Here's how the part is built. I have some questions about the finished solid (model axes, mm). Face numbers are marked on the shaded views. A direction names the side the tool comes from. Round coordinates to 2 decimals unless told otherwise and drop trailing zeros. Loops run counter-clockwise (first coordinate to the right, second up) from the corner with the lowest first, then second, coordinate; pieces in that order, holes last. Notation, with made-up numbers: M 68,12.25 L 75,12.25 A14 ccw 75,22.25 Z; hole C -30,26 d3. An arc over 180 degrees is marked long. One line per question, with ' | ' between items. Start each with the question number.
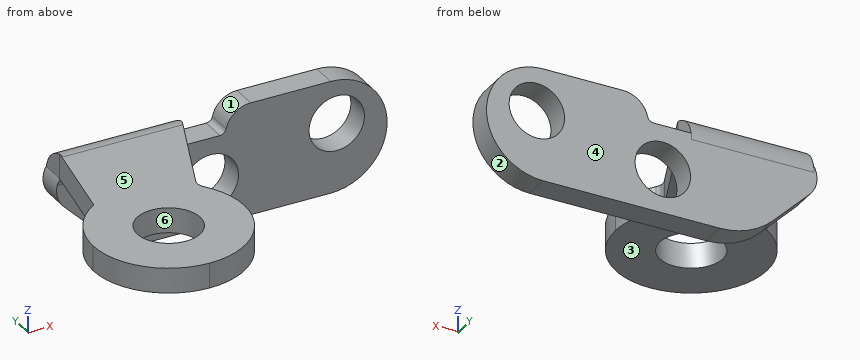
```python
from build123d import *

# Parameters (mm, degrees)
F1_DEPTH     = 2
F2_D         = 4.4
F3_W         = 13.8216872486
F3_H         = 2
F4_DEPTH     = 20.5
F5_R         = 2.5
F6_DEPTH     = 25
F7_R         = 1
F8_T4_DEPTH  = 12.2216872486
F8_T10_DEPTH = 12.2216872486
F8_S11_R     = 2
F8_T12_DEPTH = 8
F10_DEPTH    = 9.7216872486


# Not quite as in the source:
# - a fillet or chamfer that OpenCascade refuses, or shapes differently, is made with other operations: its cross-section is extruded or revolved along the edge and cut away or added


with BuildPart() as f1:
    # F0 (on Front) → F1 (new body)
    with BuildSketch(Plane.XZ):
        with BuildLine():
            Line((-5.5351668461, -4.5), (8.4648331539, -4.5))
            ThreePointArc((8.4648331539, -4.5), (12.9648331539, 0), (8.4648331539, 4.5))
            Line((8.4648331539, 4.5), (2.1292536968, 4.5))
            ThreePointArc((2.1292536968, 4.5), (0.8745117295, 4.0574410408), (0.1750670613, 2.9256225954))
            ThreePointArc((0.1750670613, 2.9256225954), (0.0002058943, 2.6426679841), (-0.3134795975, 2.5320282443))
            Line((-0.3134795975, 2.5320282443), (-13.0351668461, 2.5320282443))
            ThreePointArc((-13.0351668461, 2.5320282443), (-13.2536814771, 1.2929397336), (-12.6890072408, 0.1685590205))
            Line((-12.6890072408, 0.1685590205), (-9.7778075332, -2.7426406871))
            ThreePointArc((-9.7778075332, -2.7426406871), (-7.8312674403, -4.0432771951), (-5.5351668461, -4.5))
        make_face()
    extrude(amount=F1_DEPTH)

    # F2 (through all)
    with Locations(Plane(origin=(0, 0, 0), x_dir=(1, 0, 0), z_dir=(0, 1, 0))):
        with Locations((-1.0351668461, 1), (8.9648331539, -1)):
            Hole(F2_D / 2)

    # F3 (on face) → F4 (join)
    with BuildSketch(Plane(origin=(0, 0, 0), x_dir=(-1, 0, 0), z_dir=(0, 1, 0))):
        with Locations((10.2243232218, 3.5320282443)):
            Rectangle(F3_W, F3_H)
    extrude(amount=-F4_DEPTH)

    # F5 (on face) → F6 (cut)
    with BuildSketch(Plane(origin=(0, 0, 2.5320282443), x_dir=(1, 0, 0), z_dir=(0, 0, -1))):
        with BuildLine():
            Line((-6.7216205274, 10.43544481), (-3.3134795975, 2))
            Line((-3.3134795975, 2), (-3.3134795975, 20.5))
            Line((-3.3134795975, 20.5), (-11.1351668461, 20.5))
            ThreePointArc((-11.1351668461, 20.5), (-6.892526159, 18.7426406871), (-5.1351668461, 14.5))
            ThreePointArc((-5.1351668461, 14.5), (-5.5458342423, 12.3184040145), (-6.7216205274, 10.43544481))
        make_face()
        with BuildLine():
            Line((-17.1351668461, 20.5), (-17.1351668461, 14.5))
            ThreePointArc((-17.1351668461, 14.5), (-15.3778075332, 18.7426406871), (-11.1351668461, 20.5))
            Line((-11.1351668461, 20.5), (-17.1351668461, 20.5))
        make_face()
        with BuildLine():
            Line((-17.1351668461, 0), (-13.0351668461, 0))
            Line((-13.0351668461, 0), (-13.0351668461, 2))
            Line((-13.0351668461, 2), (-14.3454662645, 9.4310772699))
            ThreePointArc((-14.3454662645, 9.4310772699), (-16.3916769293, 11.6070600171), (-17.1351668461, 14.5))
            Line((-17.1351668461, 14.5), (-17.1351668461, 0))
        make_face()
        with Locations((-11.1351668461, 14.5)):
            Circle(F5_R)
    extrude(amount=-F6_DEPTH, mode=Mode.SUBTRACT)

    # F7
    f7_edges = [f1.edges().sort_by_distance(p)[0] for p in [
        (-6.721621, -10.435445, 3.532028),
    ]]
    fillet(f7_edges, radius=F7_R)

    # F8: fillet of radius 0.5 on 1 edges, made by hand


with BuildPart() as f8_tool2:
    # F8_s3 → F8_t4 (new body)
    with BuildSketch(Plane.YZ.offset(-2.0634795975)):
        with BuildLine():
            ThreePointArc((-2.5, 2.5320282443), (-2.1464466094, 2.3855816349), (-2, 2.0320282443))
            Line((-2, 2.0320282443), (-2, 2.5320282443))
            Line((-2, 2.5320282443), (-2.5, 2.5320282443))
        make_face()
    extrude(amount=-F8_T4_DEPTH)

    split(bisect_by=Plane(origin=(-2.1538403044, 0.8702079692, 0), x_dir=(0, 0, 1), z_dir=(-0.9271838546, 0.3746065934, 0)), keep=Keep.TOP)

    split(bisect_by=Plane(origin=(-12.3000883277, 2.1688374373, 0), x_dir=(0, 0, 1), z_dir=(0.984807753, -0.1736481777, 0)), keep=Keep.TOP)


with BuildPart() as f1_1:
    add(f1.part)

    # F8_t1: union F8_tool2
    add(f8_tool2.part)


with BuildPart() as f8_tool8:
    # F8_s9 → F8_t10 (new body)
    with BuildSketch(Plane.YZ.offset(-2.0634795975)):
        with BuildLine():
            ThreePointArc((-2.5, 2.5320282443), (-2.1464466094, 2.3855816349), (-2, 2.0320282443))
            Line((-2, 2.0320282443), (-2, 2.5320282443))
            Line((-2, 2.5320282443), (-2.5, 2.5320282443))
        make_face()
    extrude(amount=-F8_T10_DEPTH)

    # F8_s11 → F8_t12 (intersect, symmetric)
    with BuildSketch(Plane.XZ.offset(2.2)):
        with Locations((-11.2747936785, 1.5827725829)):
            Circle(F8_S11_R)
    extrude(amount=F8_T12_DEPTH, both=True, mode=Mode.INTERSECT)


with BuildPart() as f1_2:
    add(f1_1.part)

    # F8_t7: union F8_tool8
    add(f8_tool8.part)

    # F9 (on face) → F10 (cut, through all)
    with BuildSketch(Plane(origin=(-13.0351668461, 0, 0), x_dir=(0, -1, 0), z_dir=(-1, 0, 0))):
        with BuildLine():
            Line((2.5, 4.5320282443), (2, 4.5320282443))
            Line((2, 4.5320282443), (0, 4.5320282443))
            Line((0, 4.5320282443), (0, 2.5320282443))
            Line((0, 2.5320282443), (0, 2.0320282443))
            ThreePointArc((0, 2.0320282443), (0.732233047, 3.7997951973), (2.5, 4.5320282443))
        make_face()
    extrude(amount=-F10_DEPTH, mode=Mode.SUBTRACT)


solid = f1_2.part
```
1) Imagine slicing it at B-B (y = -4.5). Write out the boundary of the cut face in (x, z).
2) Imagine slicing it at A-A (z = -0.25). Write out the boundary of the cut face in (x, y), then the cut area to 3 significant figures.
3) We'd pull the mould along Y, two halves only. Please class the marked faces 4, 5 and 6: pulls with the +Y half, pulls with the -Y half, needs draft (parallel to the pull), parting line crosses it, or undercut.
4) Imagine slicing it at C-C (z = -4). Write out the boundary of the cut face in (x, y).
5) Please list where these lines run through material, in increasing order: L1, parallel to Z at x = -6, y = -6.75; L2, parallel to X at y = -14.5, z = 3.9; L3, parallel to Y at x = -5, z = 1.25. Write a range as from..to.
6) For the marked faces 1, 2 and 3, which set-ups out of +Z, -Z, +X, -X, +Y, -Y let a thin tool reach every point of the face, with its end or its side?
7) I'm going to push flat-ended pins straight in: pin 1 Ø2 at (x, y) = (-1, -1.5) entering from +Z; pin 2 Ø1 at (x, z) = (6.5, -1.5) entering from -Y; pin 3 Ø0.6 at (y, z) = (-1, 3) entering from -X. Where does each tip first touch, or does it pass through?
Results are:
1) outline: M -13.48,2.53 L -4.32,2.53 L -4.32,4.53 L -13.48,4.53 Z
2) outline: M -12.27,-2 L -3.1,-2 L -3.1,0 L -12.27,0 Z; M 1.03,-2 L 7.15,-2 L 7.15,0 L 1.03,0 Z; M 10.78,-2 L 12.96,-2 L 12.96,0 L 10.78,0 Z | area: 34.9 mm²
3) face 4: pulls with the +Y half | face 5: needs draft | face 6: undercut
4) outline: M -7.93,-2 L 10.53,-2 L 10.53,0 L -7.93,0 Z
5) L1: 2.53..4.53 | L2: -17.14..-13.64, -8.64..-5.14 | L3: -2..0
6) face 1: +Z, +Y, -Y | face 2: +X, +Y, -Y | face 3: -Z, +X, -X, -Y
7) pin 1: z = 2.64 | pin 2: y = -2 | pin 3: x = -13.04
